The model under review builds one solid part; all positions refer to its coordinate system, in mm. Face numbers are marked on the shaded views. Round coordinates to 2 decimals unless told otherwise and drop trailing zeros. Write each loop counter-clockwise with the first axis right and the second up, starting at its lowest first coordinate (ties: lowest second). Pieces come first, ordered by that corner, then holes. Notation, with made-up numbers: M -10,40.5 L -5,40.5 A23 ccw -5,65.5 Z; hole C -10,-12 d9. An arc over 180 degrees is marked long. One line per item, written item: value. Start each with the question number.
1) Take a section at C-C, the plane z = -80. Write out the cut boundary in (x, y) (1 decimal), and give its area (3 significant figures).
2) For P1, Ø3, axis at y = -17, z = -163.5, coming from the -X side; P2, Ø4, axis at y = 14, z = 104.5, coming from the +X side; P3, Ø12, axis at y = -7.5, z = -146.5, coming from the -X side; P4, Ø20, axis at x = -14, y = -4, coming from the +Z side, all flat-tipped, find the tip position at first contact; note any pin that passes through.
3) Take a section at D-D, the plane z = 121. Write out the cut boundary in (x, y).
4) Wall thickness on probe 1 along Y at (x, z) = (0, -61); probe 2 along Y at (x, z) = (0, 126); probe 3 along X at (y, z) = (1, 79): over which ranges is each line inside the solid? List them lowest first.
5) Mouldability with a two-part tool opening along X and no side actions: class the marked faces 1 and 2 as +X half, -X half, draft (parallel to the pull), parting line (faces both ways), or undercut.
from build123d import *

# Parameters (mm, degrees)
SKETCH3_R           = 33.3375
SKETCH3_R_2         = 29.3751
BOSS_EXTRUDE1_DEPTH = 217.325
SKETCH4_R           = 33.3375
SKETCH4_R_2         = 31.75
CUT_EXTRUDE1_DEPTH  = 102.35


with BuildPart() as part:
    # Sketch3 → Boss-Extrude1 (new, symmetric)
    with BuildSketch(Plane.XY):
        Circle(SKETCH3_R)
        Circle(SKETCH3_R_2, mode=Mode.SUBTRACT)
    extrude(amount=BOSS_EXTRUDE1_DEPTH, both=True)

    # Sketch5 → Cut-Revolve1 (revolve, cut)
    with BuildSketch(Plane(origin=(0, 0, 0), x_dir=(0, 0, -1), z_dir=(1, 0, 0)), mode=Mode.PRIVATE) as cut_revolve1_sk:
        Polygon((-217.325, 30.8375), (-215.881624327, 33.3375), (-217.325, 33.3375), align=None)
    revolve(cut_revolve1_sk.sketch.rotate(Axis((0, 0, 0), (0, 0, 1)), 90), axis=Axis((0, 0, 0), (0, 0, 1)), mode=Mode.SUBTRACT)

    # Sketch4 → Cut-Extrude1 (cut)
    with BuildSketch(Plane.XY.offset(217.325)):
        Circle(SKETCH4_R)
        Circle(SKETCH4_R_2, mode=Mode.SUBTRACT)
    extrude(amount=-CUT_EXTRUDE1_DEPTH, mode=Mode.SUBTRACT)


solid = part.part
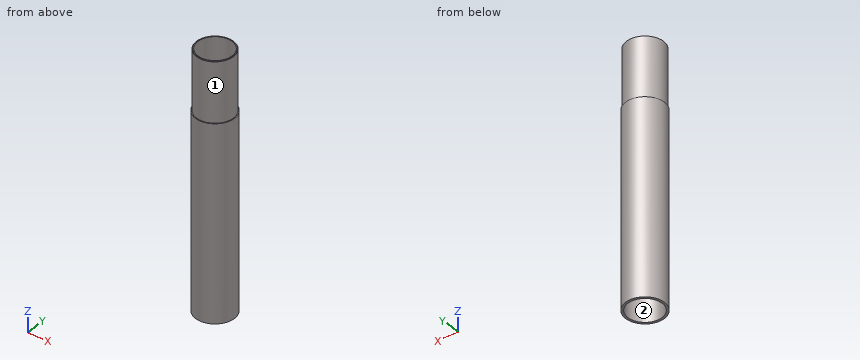
Checked values:
1. outline: C 0,0 d66.7; hole C 0,0 d58.8
1. area: 781 mm2
2. P1: stops at x = -29.52
2. P2: stops at x = 31.1
2. P3: stops at x = -33.3
2. P4: passes through
3. outline: C 0,0 d63.5; hole C 0,0 d58.75
4. probe 1: y = -33.34 to -29.38, 29.38 to 33.34
4. probe 2: y = -31.75 to -29.38, 29.38 to 31.75
4. probe 3: x = -33.32 to -29.36, 29.36 to 33.32
5. face 1: parting line
5. face 2: undercut
